Design review of the part built by this model. Coordinates are the model's own, in mm. A direction names the side the tool comes from. Give positions to 0.01 mm unless a question says otherwise; leave off trailing zeros. Order: outer loops, then holes, each group sorted by start corner. A loop starts at its lowest first (then second) coordinate and runs counter-clockwise, first axis right, second up. Notation, with made-up numbers: M 26,13 L 71,13 A19 ccw 71,22 Z; hole C 73,-18.5 d7. An arc over 180 degrees is marked long. Put each result on its own line as item: value. Start each with the question number.
from build123d import *

# Parameters (mm, degrees)
AUFSATZ_LINEAR_AUSTRAGEN1_DEPTH      = 720
AUFSATZ_LINEAR_AUSTRAGEN1_DEPTH_BACK = 720
LINEARES_MUSTER1_COUNT               = 15
LINEARES_MUSTER1_PITCH               = 100
LINEARES_MUSTER2_COUNT               = 15
LINEARES_MUSTER2_PITCH               = 100


with BuildPart() as part:
    # Skizze1 → Aufsatz-Linear austragen1 (new, two sides: drawn at the far end of the back side and taken through both)
    with BuildSketch(Plane.XY.offset(-AUFSATZ_LINEAR_AUSTRAGEN1_DEPTH_BACK)):
        Polygon((0, 0), (0, 35), (5, 35), (5, 5), (35, 5), (35, 0), align=None)
    extrude(amount=AUFSATZ_LINEAR_AUSTRAGEN1_DEPTH + AUFSATZ_LINEAR_AUSTRAGEN1_DEPTH_BACK)

    # Skizze2 → M5 Gewindebohrung1 (revolve, cut)
    with BuildSketch(Plane(origin=(15, 0, 700), x_dir=(0, 0, -1), z_dir=(1, 0, 0))):
        Polygon((0, 0), (0, 15.2618073), (2.1, 14), (2.1, 0), align=None)
    m5_gewindebohrung1 = revolve(axis=Axis((15, -6.35, 700), (0, 1, 0)), mode=Mode.SUBTRACT)

    # Lineares Muster1: M5 Gewindebohrung1 ×15
    with Locations(*[(0, 0, -i * LINEARES_MUSTER1_PITCH) for i in range(1, LINEARES_MUSTER1_COUNT)]):
        add(m5_gewindebohrung1, mode=Mode.SUBTRACT)

    # Skizze4 → M5 Gewindebohrung2 (revolve, cut)
    with BuildSketch(Plane(origin=(0, 15, 700), x_dir=(0, 0, 1), z_dir=(0, 1, 0))):
        Polygon((0, 0), (0, 15.2618073), (2.1, 14), (2.1, 0), align=None)
    m5_gewindebohrung2 = revolve(axis=Axis((-6.35, 15, 700), (1, 0, 0)), mode=Mode.SUBTRACT)

    # Lineares Muster2: M5 Gewindebohrung2 ×15
    with Locations(*[(0, 0, -i * LINEARES_MUSTER2_PITCH) for i in range(1, LINEARES_MUSTER2_COUNT)]):
        add(m5_gewindebohrung2, mode=Mode.SUBTRACT)


solid = part.part
1. To check wall thickness, follow probe 1 along X at (y, z) = (2.55, -300); probe 2 along X at (y, z) = (14.5, 326). State the ranges of each line that lie inside material, in increasing order.
2. Insertion check: pin 1 (6.5 mm diameter, centred on y = 15, z = -500, fed in from +X); pin 2 (5.5 mm diameter, centred on x = 15, z = -600, fed in from +Y). Each pin has a flat end and moves straight along its axis. Give the tip position at first contact, or say it passes through.
3. Machinability: for faces 1 (the flat face through (5, 20, -10)), 2 (the flat face through (0, 17, -10)), which of the approach directions +Z, -Z, +X, -X, +Y, -Y give a long, thin tool a straight path to every point of the face, cutting with its end or side? Answer none if there is none.
4. Consider section A-A on z = -524.5. Give the boundary of the cut face in (x, y).
Returned:
1. probe 1: x = 0 to 12.9, 17.1 to 35
1. probe 2: x = 0 to 5
2. pin 1: stops at x = 5
2. pin 2: stops at y = 5
3. face 1: +Z, -Z, +X, +Y
3. face 2: +Z, -Z, -X, +Y, -Y
4. outline: M 0,0 L 35,0 L 35,5 L 5,5 L 5,35 L 0,35 Z
